Geometry check sheet. Reference: drawing and pictorial views, mm from the part's lowest x, y, z. Coordinates: 2 decimals unless noted, no trailing zeros. Loops run counter-clockwise (first coordinate to the right, second up) from the corner with the lowest first, then second, coordinate; pieces in that order, holes last.
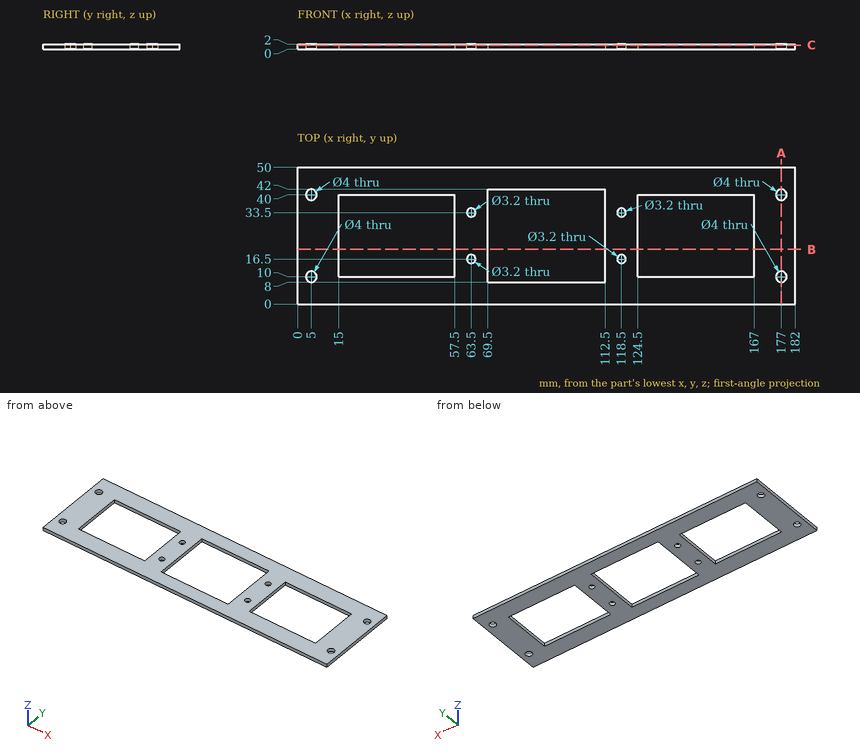
1) Material ranges on probe 1 along Y at (x, z) = (177, 1.1); probe 2 along X at (y, z) = (27, 0.4); probe 3 along Y at (x, z) = (63.5, 0.55), recorded low to high.
Data:
probe 1: y = 0 to 8, 12 to 38, 42 to 50
probe 2: x = 0 to 15, 57.5 to 69.5, 112.5 to 124.5, 167 to 182
probe 3: y = 0 to 14.9, 18.1 to 31.9, 35.1 to 50
2) Section check C-C on z = 1.6. Count the separate pieces of the cut face and the enclosed holes in it, and give its area (3 significant figures).
Data:
separate pieces: 1
enclosed holes: 11
area: 5,010 mm2
3) Section check B-B on y = 20. Record the cut outline in (x, z).
Data:
outline: (0, 0) - (15, 0) - (15, 2) - (0, 2) - close; (57.5, 0) - (69.5, 0) - (69.5, 2) - (57.5, 2) - close; (112.5, 0) - (124.5, 0) - (124.5, 2) - (112.5, 2) - close; (167, 0) - (182, 0) - (182, 2) - (167, 2) - close
4) Section check A-A on x = 177. Record the cut outline in (y, z).
Data:
outline: (0, 0) - (8, 0) - (8, 2) - (0, 2) - close; (12, 0) - (38, 0) - (38, 2) - (12, 2) - close; (42, 0) - (50, 0) - (50, 2) - (42, 2) - close
